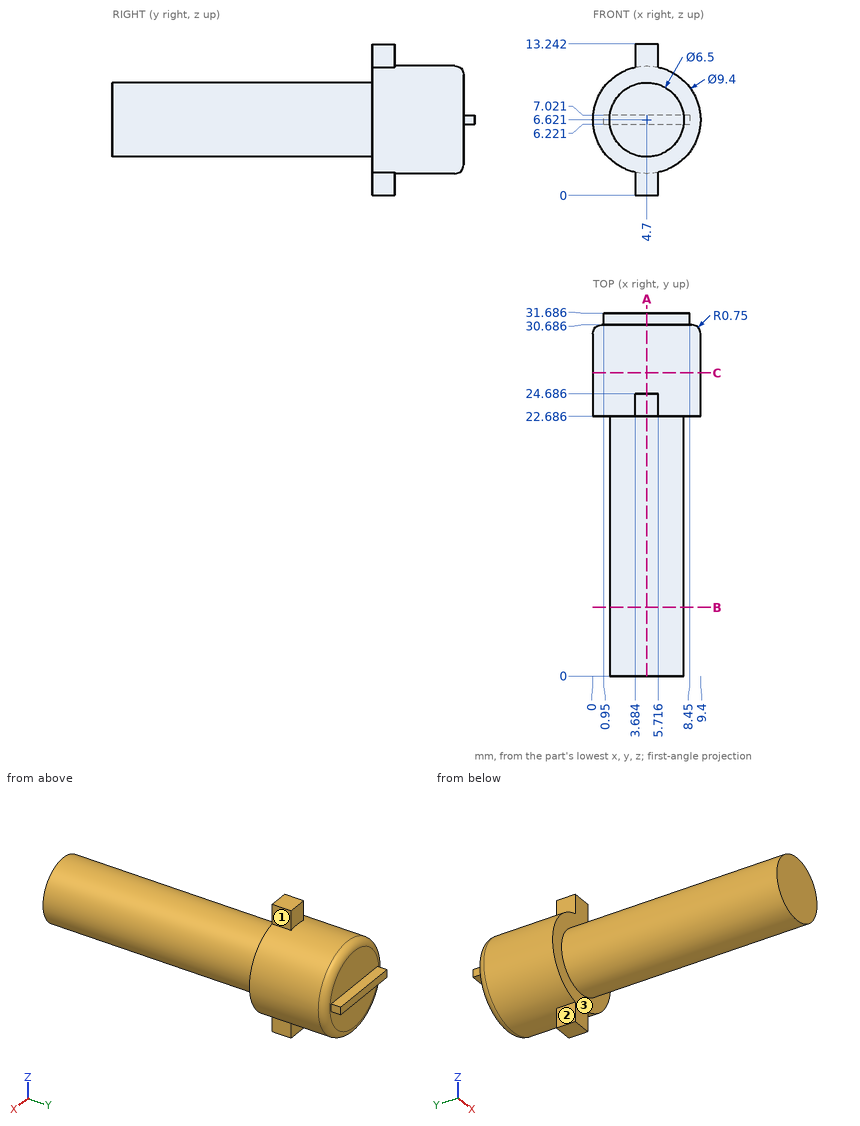
The drawing under review shows one solid part. Ordinate dimensions are in mm from its lowest x, y, z. A direction names the side the tool comes from. Give positions to 0.01 mm unless a question says otherwise; leave off trailing zeros. Order: outer loops, then holes, each group sorted by start corner. A loop starts at its lowest first (then second) coordinate and runs counter-clockwise, first axis right, second up. Notation, with made-up numbers: M 17.25,48.25 L 59.25,48.25 A25 ccw 59.25,70.25 Z; hole C 59.25,34.5 d2. An arc over 180 degrees is marked long. Answer in a Markdown table with one row per item. Add a question column.
1. To check wall thickness, follow line 1 along Y through (x, z) = (4.25, 2.75); line 2 along Y through (x, z) = (6.5, 9); line 3 along Z through (x, y) = (4.25, 2). State the ranges of each line that lie inside material, in increasing order.
2. Add section C-C on y = 26.5. State the section outline as (x, z) points.
3. Add section A-A on x = 4.7. State the section outline as (y, z) points.
4. For pin 1 Ø6 at (y, z) = (8, 8.5) entering from -X; pin 2 Ø1 at (y, z) = (18.5, 8) entering from +X; pin 3 Ø4 at (x, y) = (7.5, 27.5) entering from +Z, all flat-tipped, find the tip position at first contact; note any pin that passes through.
5. Machinability: for the marked faces 1, 2 and 3, which of the approach directions +Z, -Z, +X, -X, +Y, -Y give a long, thin tool a straight path to every point of the face, cutting with its end or side? Answer none if there is none.
6. Add section B-B on y = 6. State the section outline as (x, z) points.
The answers:
| question | item | result |
|---|---|---|
| 1 | line 1 | 22.69 to 30.69 |
| 1 | line 2 | 0 to 30.69 |
| 1 | line 3 | 3.4 to 9.84 |
| 2 | outline | C 4.7,6.62 d9.4 |
| 3 | outline | M 0,3.37 L 22.69,3.37 L 22.69,0 L 24.69,0 L 24.69,1.92 L 29.94,1.92 A0.75 ccw 30.69,2.67 L 30.69,6.22 L 31.69,6.22 L 31.69,7.02 L 30.69,7.02 L 30.69,10.57 A0.75 ccw 29.94,11.32 L 24.69,11.32 L 24.69,13.24 L 22.69,13.24 L 22.69,9.87 L 0,9.87 Z |
| 4 | pin 1 | x = 1.45 |
| 4 | pin 2 | x = 7.83 |
| 4 | pin 3 | z = 11.25 |
| 5 | face 1 | +Z, +X, +Y, -Y |
| 5 | face 2 | -Z, -X, +Y, -Y |
| 5 | face 3 | -Y |
| 6 | outline | C 4.7,6.62 d6.5 |
